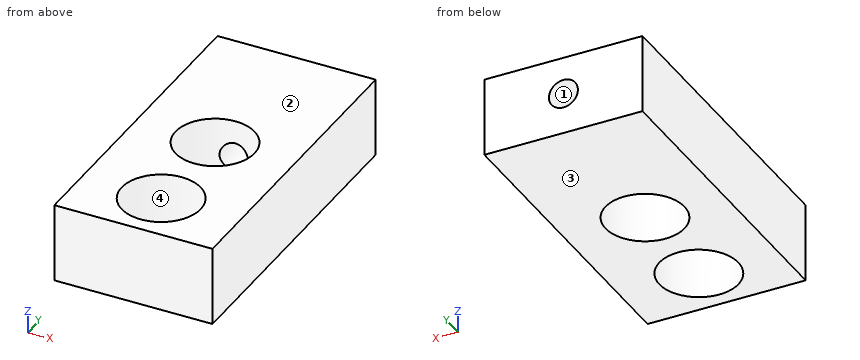
from build123d import *

# Parameters (mm, degrees)
F0_W     = 12.7
F0_H     = 25.4
F0_R     = 3.175
F1_DEPTH = 6.35
F2_R     = 1.162114
F3_DEPTH = 10.16


with BuildPart() as f1:
    # F0 (on Top) → F1 (new body)
    with BuildSketch(Plane.XY):
        Rectangle(F0_W, F0_H)
        with Locations((0, -8.382)):
            Circle(F0_R, mode=Mode.SUBTRACT)
        Circle(F0_R, mode=Mode.SUBTRACT)
    extrude(amount=F1_DEPTH)

    # F2 (on face) → F3 (cut)
    with BuildSketch(Plane(origin=(0, 12.7, 0), x_dir=(-1, 0, 0), z_dir=(0, 1, 0))):
        with Locations((0, 3.320315)):
            Circle(F2_R)
    extrude(amount=-F3_DEPTH, mode=Mode.SUBTRACT)


solid = f1.part
Can you work these out from the model? Positions are in its coordinate system, mm. Face numbers are marked on the shaded views. Coordinates: 2 decimals unless noted, no trailing zeros. Order: outer loops, then holes, each group sorted by start corner. A loop starts at its lowest first (then second) coordinate and runs counter-clockwise, first axis right, second up. Notation, with made-up numbers: M 55.25,-19 L 96.25,-19 A18 ccw 96.25,-7 Z; hole C -2.5,-19 d9. An arc over 180 degrees is marked long. Answer as CSV lines item,"result".
(1) Suppose I cut it at D-D on z = 5.25. Please give me the cut outline in (x, y) (3 decimals).
Geometry check:
outline,"M -6.35,-12.7 L 6.35,-12.7 L 6.35,12.7 L -6.35,12.7 Z; hole C 0,-8.382 d6.35; hole C 0,0 d6.35"
(2) If we mould it in two halves opening along Z, with no side actions, what happens to the marked faces 1, 2, 3 and 4? For each: released by +Z, released by -Z, zero draft, split by the parting line, or undercut.
Geometry check:
face 1,"undercut"
face 2,"released by +Z"
face 3,"released by -Z"
face 4,"zero draft"
(3) I'm going to push a flat-ended pin straight in: pin 1 (1 mm diameter, centred on x = 1.5, y = -9.5, fed in from -Z). Where does the tip first touch, or does it pass through?
Geometry check:
pin 1,"through"
(4) Suppose I cut it at C-C on z = 2.75. Please give me the cut outline in (x, y) (3 decimals).
Geometry check:
outline,"M -6.35,-12.7 L 6.35,-12.7 L 6.35,12.7 L 1.013,12.7 L 1.013,3.009 A3.175 cw long -1.013,3.009 L -1.013,12.7 L -6.35,12.7 Z; hole C 0,-8.382 d6.35"
(5) Please list where these lines run through material, in increasing order: L1, parallel to Y at x = 0, z = 5 (3 decimals); L2, parallel to Z at x = 0, y = 6.75; L3, parallel to Y at x = 0, z = 4 (3 decimals).
Geometry check:
L1,"-12.7 to -11.557, -5.207 to -3.175, 3.175 to 12.7"
L2,"0 to 2.16, 4.48 to 6.35"
L3,"-12.7 to -11.557, -5.207 to -3.175"
(6) Suppose I cut it at A-A on y = 0. Please give me the cut outline in (x, z) (3 decimals).
Geometry check:
outline,"M -6.35,0 L -3.175,0 L -3.175,6.35 L -6.35,6.35 Z; M 3.175,0 L 6.35,0 L 6.35,6.35 L 3.175,6.35 Z"
(7) Suppose I cut it at B-B on x = 0. Please give me the cut outline in (y, z) (3 decimals).
Geometry check:
outline,"M -12.7,0 L -11.557,0 L -11.557,6.35 L -12.7,6.35 Z; M -5.207,0 L -3.175,0 L -3.175,6.35 L -5.207,6.35 Z; M 3.175,0 L 12.7,0 L 12.7,2.158 L 3.175,2.158 Z; M 3.175,4.482 L 12.7,4.482 L 12.7,6.35 L 3.175,6.35 Z"
